Read the model definition and answer for the solid it produces. Units are mm, in the model's axes. A direction names the side the tool comes from. Give positions to 0.01 mm unless a question says otherwise; leave off trailing zeros. Write each loop counter-clockwise with the first axis right and the second up, starting at its lowest first coordinate (ties: lowest second). Pieces come first, ordered by that corner, then holes. Notation, with made-up numbers: (-10, -37.75) - (37, -37.75) arc R29 cw to (37, -9.75) - close; hole circle Ø10 at (80, 43.5). An arc over 180 degrees is marked (long way). Answer as CSV lines item,"result".
```python
from build123d import *

# Parameters (mm, degrees)
PAD_DEPTH       = 10
SKETCH001_R     = 16.5
POCKET_DEPTH    = 8
SKETCH002_R     = 16.5
POCKET001_DEPTH = 8
SKETCH003_R     = 16.5
POCKET002_DEPTH = 8
SKETCH004_R     = 16.5
POCKET003_DEPTH = 8
SKETCH005_R     = 16.5
POCKET004_DEPTH = 8
SKETCH006_R     = 16.5
POCKET005_DEPTH = 8
SKETCH007_R     = 5.125
POCKET006_DEPTH = 1.15
SKETCH008_R     = 5.125
POCKET007_DEPTH = 1.15


with BuildPart() as part:
    # Sketch → Pad (new body)
    with BuildSketch(Plane.XY):
        with BuildLine():
            ThreePointArc((71.830952, -16.5), (78.374369, 12.374369), (49.5, 5.830952))
            ThreePointArc((49.5, 5.830952), (33, 17.5), (16.5, 5.830952))
            ThreePointArc((16.5, 5.830952), (-12.374369, 12.374369), (-5.830952, -16.5))
            ThreePointArc((-5.830952, -16.5), (-12.374369, -45.374369), (16.5, -38.830952))
            ThreePointArc((16.5, -38.830952), (33, -50.5), (49.5, -38.830952))
            ThreePointArc((49.5, -38.830952), (78.374369, -45.374369), (71.830952, -16.5))
        make_face()
        with BuildLine():
            ThreePointArc((5.830952, -16.5), (7.543698, -15.790586), (9.171788, -14.903969))
            ThreePointArc((9.171788, -14.903969), (9, -16.5), (9.171788, -18.096031))
            ThreePointArc((9.171788, -18.096031), (7.543698, -17.209414), (5.830952, -16.5))
        make_face(mode=Mode.SUBTRACT)
        with BuildLine():
            ThreePointArc((47.903969, -9.171788), (48.790586, -7.543698), (49.5, -5.830952))
            ThreePointArc((49.5, -5.830952), (50.209414, -7.543698), (51.096031, -9.171788))
            ThreePointArc((51.096031, -9.171788), (49.5, -9), (47.903969, -9.171788))
        make_face(mode=Mode.SUBTRACT)
        with BuildLine():
            ThreePointArc((18.096031, -23.828212), (17.209414, -25.456302), (16.5, -27.169048))
            ThreePointArc((16.5, -27.169048), (15.790586, -25.456302), (14.903969, -23.828212))
            ThreePointArc((14.903969, -23.828212), (16.5, -24), (18.096031, -23.828212))
        make_face(mode=Mode.SUBTRACT)
        with BuildLine():
            ThreePointArc((47.903969, -23.828212), (49.5, -24), (51.096031, -23.828212))
            ThreePointArc((51.096031, -23.828212), (50.209414, -25.456302), (49.5, -27.169048))
            ThreePointArc((49.5, -27.169048), (48.790586, -25.456302), (47.903969, -23.828212))
        make_face(mode=Mode.SUBTRACT)
        with BuildLine():
            ThreePointArc((14.903969, -9.171788), (15.790586, -7.543698), (16.5, -5.830952))
            ThreePointArc((16.5, -5.830952), (17.209414, -7.543698), (18.096031, -9.171788))
            ThreePointArc((18.096031, -9.171788), (16.5, -9), (14.903969, -9.171788))
        make_face(mode=Mode.SUBTRACT)
        with BuildLine():
            ThreePointArc((23.828212, -18.096031), (24, -16.5), (23.828212, -14.903969))
            ThreePointArc((23.828212, -14.903969), (25.456302, -15.790586), (27.169048, -16.5))
            ThreePointArc((27.169048, -16.5), (25.456302, -17.209414), (23.828212, -18.096031))
        make_face(mode=Mode.SUBTRACT)
        with BuildLine():
            ThreePointArc((42.171788, -18.096031), (40.543698, -17.209414), (38.830952, -16.5))
            ThreePointArc((38.830952, -16.5), (40.543698, -15.790586), (42.171788, -14.903969))
            ThreePointArc((42.171788, -14.903969), (42, -16.5), (42.171788, -18.096031))
        make_face(mode=Mode.SUBTRACT)
        with BuildLine():
            ThreePointArc((56.828212, -18.096031), (57, -16.5), (56.828212, -14.903969))
            ThreePointArc((56.828212, -14.903969), (58.456302, -15.790586), (60.169048, -16.5))
            ThreePointArc((60.169048, -16.5), (58.456302, -17.209414), (56.828212, -18.096031))
        make_face(mode=Mode.SUBTRACT)
    extrude(amount=PAD_DEPTH)

    # Sketch001 (on Face32 of Pad) → Pocket (cut)
    with BuildSketch(Plane.XY.offset(10)):
        Circle(SKETCH001_R)
    extrude(amount=-POCKET_DEPTH, mode=Mode.SUBTRACT)

    # Sketch002 (on Face5 of Pocket) → Pocket001 (cut)
    with BuildSketch(Plane.XY.offset(10)):
        with Locations((33, 0)):
            Circle(SKETCH002_R)
    extrude(amount=-POCKET001_DEPTH, mode=Mode.SUBTRACT)

    # Sketch003 (on Face5 of Pocket001) → Pocket002 (cut)
    with BuildSketch(Plane.XY.offset(10)):
        with Locations((66, 0)):
            Circle(SKETCH003_R)
    extrude(amount=-POCKET002_DEPTH, mode=Mode.SUBTRACT)

    # Sketch004 (on Face5 of Pocket002) → Pocket003 (cut)
    with BuildSketch(Plane.XY.offset(10)):
        with Locations((0, -33)):
            Circle(SKETCH004_R)
    extrude(amount=-POCKET003_DEPTH, mode=Mode.SUBTRACT)

    # Sketch005 (on Face5 of Pocket003) → Pocket004 (cut)
    with BuildSketch(Plane.XY.offset(10)):
        with Locations((33, -33)):
            Circle(SKETCH005_R)
    extrude(amount=-POCKET004_DEPTH, mode=Mode.SUBTRACT)

    # Sketch006 (on Face5 of Pocket004) → Pocket005 (cut)
    with BuildSketch(Plane.XY.offset(10)):
        with Locations((66, -33)):
            Circle(SKETCH006_R)
    extrude(amount=-POCKET005_DEPTH, mode=Mode.SUBTRACT)

    # Sketch007 (on Face4 of Pocket005) → Pocket006 (cut)
    with BuildSketch(Plane(origin=(0, 0, 0), x_dir=(1, 0, 0), z_dir=(0, 0, -1))):
        with Locations((16.5, 16.5)):
            Circle(SKETCH007_R)
    extrude(amount=-POCKET006_DEPTH, mode=Mode.SUBTRACT)

    # Sketch008 (on Face4 of Pocket006) → Pocket007 (cut)
    with BuildSketch(Plane(origin=(0, 0, 0), x_dir=(1, 0, 0), z_dir=(0, 0, -1))):
        with Locations((49.5, 16.5)):
            Circle(SKETCH008_R)
    extrude(amount=-POCKET007_DEPTH, mode=Mode.SUBTRACT)


solid = part.part
```
(1) A cutting plane is placed at A-A (x = -7). Write down the section's boundary in (y, z).
Worked out:
outline,"(-49.04, 0) - (-16.96, 0) - (-16.96, 10) - (-18.06, 10) - (-18.06, 2) - (-47.94, 2) - (-47.94, 10) - (-49.04, 10) - close; (-16.04, 0) - (16.04, 0) - (16.04, 10) - (14.94, 10) - (14.94, 2) - (-14.94, 2) - (-14.94, 10) - (-16.04, 10) - close"
(2) A cutting plane is placed at B-B (y = -43). Write down the section's boundary in (x, z).
Worked out:
outline,"(-14.36, 0) - (14.36, 0) - (14.36, 10) - (13.12, 10) - (13.12, 2) - (-13.12, 2) - (-13.12, 10) - (-14.36, 10) - close; (18.64, 0) - (47.36, 0) - (47.36, 10) - (46.12, 10) - (46.12, 2) - (19.88, 2) - (19.88, 10) - (18.64, 10) - close; (51.64, 0) - (80.36, 0) - (80.36, 10) - (79.12, 10) - (79.12, 2) - (52.88, 2) - (52.88, 10) - (51.64, 10) - close"
(3) Each of these flat-tipped pins is pushed along its axis until it touches: P1, Ø2, axis at x = 51, y = -18, coming from the -Z side; P2, Ø10, axis at x = 30, y = 0, coming from the +Z side; P3, Ø6, axis at x = 59, z = 4.5, coming from the -Y side; P4, Ø8, axis at x = 51.5, y = -16.5, coming from the -Z side. Where does it stop, or does it pass through?
Worked out:
P1,"stops at z = 1.15"
P2,"stops at z = 2"
P3,"stops at y = -50.04"
P4,"stops at z = 0"
(4) For faces 3 (the flat face through (32, -16, 0)), 4 (the cylindrical face through (77.276, -45.046, 6.056)), 5 (the cylindrical face through (12.433, -13.382, 0.567)), determine the directions among +Z, -Z, +X, -X, +Y, -Y from which every point of the face is accessible in a straight line to the end or side of a thin tool.
Worked out:
face 3,"-Z, +X, -X, +Y, -Y"
face 4,"+Z"
face 5,"-Z"
(5) Find the intervals of material crossed by L1, parallel to X at y = -22.5, z = 4.75; L2, parallel to X at y = -21.5, z = 3.5; L3, parallel to X at y = 9, z = 6.75, in increasing order.
Worked out:
L1,"x = -14 to -12.73, 12.73 to 20.27, 45.73 to 53.27, 78.73 to 80"
L2,"x = -13.19 to -11.83, 11.83 to 21.17, 44.83 to 54.17, 77.83 to 79.19"
L3,"x = -15.01 to -13.83, 13.83 to 15.01, 17.99 to 19.17, 46.83 to 48.01, 50.99 to 52.17, 79.83 to 81.01"
(6) The mould has two halves that part along X. Classify faces 1 (the flat face through (49, -18, 10)), 2 (the cylindrical face through (78.72, 12.02, 4.93)): +X half, -X half, draft (parallel to the pull), parting line (faces both ways), or undercut.
Worked out:
face 1,"draft"
face 2,"undercut"
